from build123d import *

# Parameters (mm, degrees)
SKETCH1_R           = 25
SKETCH1_R_2         = 2.5
BOSS_EXTRUDE1_DEPTH = 20
BOSS_EXTRUDE3_START = 14.5
BOSS_EXTRUDE3_DEPTH = 14.5
SKETCH7_R           = 15
BOSS_EXTRUDE4_DEPTH = 3
FILLET1_R           = 1


with BuildPart() as part:
    # Sketch1 → Boss-Extrude1 (new body)
    with BuildSketch(Plane(origin=(0, 0, 0), x_dir=(1, 0, 0), z_dir=(0, 1, 0))):
        with Locations(Location((0, 0, 0), (0, 0, 270))):
            Circle(SKETCH1_R)
        with Locations(Location((0, 0, 0), (0, 0, 270))):
            Circle(SKETCH1_R_2, mode=Mode.SUBTRACT)
    extrude(amount=BOSS_EXTRUDE1_DEPTH)

    # Sketch2 → Boss-Extrude3 (add)
    with BuildSketch(Plane.XZ.offset(BOSS_EXTRUDE3_START)):
        with BuildLine():
            ThreePointArc((-2, 3.464101615), (-4, 0), (-2, -3.464101615))
            ThreePointArc((-2, -3.464101615), (4, 0), (-2, 3.464101615))
        make_face()
        with BuildLine():
            ThreePointArc((-2, 1.5), (2.5, 0), (-2, -1.5))
            ThreePointArc((-2, -1.5), (-2.5, 0), (-2, 1.5))
        make_face(mode=Mode.SUBTRACT)
    extrude(amount=-BOSS_EXTRUDE3_DEPTH)

    # Sketch7 → Boss-Extrude4 (add)
    with BuildSketch(Plane.XZ):
        with Locations(Location((0, 0, 0), (0, 0, 90))):
            Circle(SKETCH7_R)
    extrude(amount=BOSS_EXTRUDE4_DEPTH)

    # Fillet1
    fillet1_edges = [part.edges().sort_by_distance(p)[0] for p in [
        (2, -3, -3.464101615),
    ]]
    fillet(fillet1_edges, radius=FILLET1_R)


solid = part.part
The listing builds one solid part. Answer for the finished solid, in the listing's coordinates (mm). A direction names the side the tool comes from. Coordinates: 2 decimals unless noted, no trailing zeros. Loops run counter-clockwise (first coordinate to the right, second up) from the corner with the lowest first, then second, coordinate; pieces in that order, holes last. Notation, with made-up numbers: (31.25, -22) -> (58.25, -22) arc R20 cw to (58.25, -3) -> close; hole circle Ø4 at (-3, -11). An arc over 180 degrees is marked (long way). Write item = value, one per line. Start each with the question number.
1) A cutting plane is placed at D-D (x = -14). Give the vertices of the cut face in (y, z), then the cut area to 3 significant figures.
2) Given pin 1 Ø4 at (x, z) = (0, 0) entering from -Y; pin 2 Ø1 at (x, z) = (-17, 11.5) entering from -Y; pin 3 Ø1.5 at (x, z) = (-0.5, 0.5) entering from +Y, each flat-ended and moving along its own axis, determine where each tip first touches the part or whether it passes through.
3) A cutting plane is placed at B-B (x = 8). Give the vertices of the cut face in (y, z).
4) A tool of negligible diameter and unlimited length cuts with its end or side. For faces 4 (the face through (0, -3, 0)), 5 (the face through (2, -14.5, 2)), 6 (the face through (0, 0, 0)), from which of +Z, -Z, +X, -X, +Y, -Y can it reach the whole face along a straight path? Write none if from no direction.
5) A cutting plane is placed at A-A (z = 0). Give the vertices of the cut face in (x, y), then the cut area to 3 significant figures.
6) The mould has two halves that part along X. Classify faces 1 (the face through (0.751, 9.86, 2.385)), 2 (the face through (7.509, 9.86, 23.846)), 3 (the face through (-5, 20, 0)): released by +X, released by -X, zero draft, split by the parting line, or undercut.
7) Straight lines are drawn through the part: line 1 (Z direction, x = 0, y = -7); line 2 (X direction, y = 12, z = 0); line 3 (Y direction, x = -5.5, z = -13). For each, find the intervals that lie inside material, in ascending order. Write a range as from..to.
8) A cutting plane is placed at C-C (y = 14). Give the vertices of the cut face in (x, z), then the cut area to 3 significant figures.
Responses:
q1.outline = (-3, -5.39) -> (0, -5.39) -> (0, -20.71) -> (20, -20.71) -> (20, 20.71) -> (0, 20.71) -> (0, 5.39) -> (-3, 5.39) -> close
q1.area = 861 mm²
q2.pin_1 = -3
q2.pin_2 = 0
q2.pin_3 = 0
q3.outline = (-3, -12.69) -> (0, -12.69) -> (0, -23.69) -> (20, -23.69) -> (20, 23.69) -> (0, 23.69) -> (0, 12.69) -> (-3, 12.69) -> close
q4.face_4 = -Y
q4.face_5 = +Z, -Z, +X, -X, -Y
q4.face_6 = +Y
q5.outline = (-25, 0) -> (-15, 0) -> (-15, -3) -> (-5, -3) arc R1 cw to (-4, -4) -> (-4, -14.5) -> (-2.5, -14.5) -> (-2.5, -3) -> (2.5, -3) -> (2.5, -14.5) -> (4, -14.5) -> (4, -4) arc R1 cw to (5, -3) -> (15, -3) -> (15, 0) -> (25, 0) -> (25, 20) -> (2.5, 20) -> (2.5, 0) -> (-2.5, 0) -> (-2.5, 20) -> (-25, 20) -> close
q5.area = 1,020 mm²
q6.face_1 = undercut
q6.face_2 = split by the parting line
q6.face_3 = zero draft
q7.line_1 = -4..-2.5, 2.5..4
q7.line_2 = -25..-2.5, 2.5..25
q7.line_3 = -3..20
q8.outline = circle Ø50 at (0, 0); hole circle Ø5 at (0, 0)
q8.area = 1,940 mm²
